Read the model definition and answer for the solid it produces. Units are mm, in the model's axes. A direction names the side the tool comes from. Give positions to 0.01 mm unless a question says otherwise; leave off trailing zeros. Write each loop counter-clockwise with the first axis right and the second up, starting at its lowest first coordinate (ties: lowest second). Pieces come first, ordered by that corner, then holes. Notation, with made-up numbers: (25.5, 14.5) -> (49.5, 14.5) arc R16 ccw to (49.5, 41.5) -> close; hole circle Ø10 at (31.25, -38). An arc over 180 degrees is marked (long way). Use a Markdown table: item, result.
from build123d import *

# Parameters (mm, degrees)
ESQUISSE14_W       = 64.629945491
ESQUISSE14_H       = 40
ESQUISSE14_R       = 1.719219897
ESQUISSE14_R_2     = 0.762879998
BOSS_EXTRU_1_DEPTH = 2
ESQUISSE15_W       = 64.629945491
ESQUISSE15_H       = 4
BOSS_EXTRU_2_DEPTH = 10


with BuildPart() as part:
    # Esquisse14 → Boss.-Extru.1 (new body)
    with BuildSketch(Plane.XY):
        with Locations((-35.198967366, -21.902230173)):
            Rectangle(ESQUISSE14_W, ESQUISSE14_H)
        with Locations((-10.253804476, -19.851102207)):
            Circle(ESQUISSE14_R, mode=Mode.SUBTRACT)
        with Locations((-9.464985935, -35.965799335)):
            Circle(ESQUISSE14_R, mode=Mode.SUBTRACT)
        with Locations((-58.998745092, -18.695161475)):
            Circle(ESQUISSE14_R, mode=Mode.SUBTRACT)
        with Locations((-60.03027703, -35.965799335)):
            Circle(ESQUISSE14_R, mode=Mode.SUBTRACT)
        with Locations((-11.973024373, -22.81882365)):
            Circle(ESQUISSE14_R_2, mode=Mode.SUBTRACT)
    extrude(amount=-BOSS_EXTRU_1_DEPTH)

    # Esquisse15 → Boss.-Extru.2 (add)
    with BuildSketch(Plane.XY):
        with Locations((-35.198967366, -10.343644154)):
            Rectangle(ESQUISSE15_W, ESQUISSE15_H)
    extrude(amount=BOSS_EXTRU_2_DEPTH)


solid = part.part
Item 1: A cutting plane is placed at C-C (y = -29). Give the vertices of the cut face in (x, z).
Return value:
| item | result |
|---|---|
| outline | (-67.51, -2) -> (-2.88, -2) -> (-2.88, 0) -> (-67.51, 0) -> close |
Item 2: A cutting plane is placed at B-B (x = -60). Give the vertices of the cut face in (y, z).
Return value:
| item | result |
|---|---|
| outline | (-41.9, -2) -> (-37.68, -2) -> (-37.68, 0) -> (-41.9, 0) -> close; (-34.25, -2) -> (-20.09, -2) -> (-20.09, 0) -> (-34.25, 0) -> close; (-17.3, -2) -> (-1.9, -2) -> (-1.9, 0) -> (-8.34, 0) -> (-8.34, 10) -> (-12.34, 10) -> (-12.34, 0) -> (-17.3, 0) -> close |
Item 3: A cutting plane is placed at A-A (x = -41.5). Give the vertices of the cut face in (y, z).
Return value:
| item | result |
|---|---|
| outline | (-41.9, -2) -> (-1.9, -2) -> (-1.9, 0) -> (-8.34, 0) -> (-8.34, 10) -> (-12.34, 10) -> (-12.34, 0) -> (-41.9, 0) -> close |
Item 4: Each of these flat-tipped pins is pushed along its axis until it touches: P1, Ø1.8, axis at x = -11.97, y = -22.82, coming from the +Z side; P2, Ø1, axis at x = -38, z = 1.5, coming from the +Y side. Where does it stop, or does it pass through?
Return value:
| item | result |
|---|---|
| P1 | z = 0 |
| P2 | y = -8.34 |
Item 5: A tool of negligible diameter and unlimited length cuts with its end or side. For faces 1 (the face through (-36, -8.344, 5)), 2 (the face through (-36, -27, 0)), 3 (the face through (-11.52, -18.69, -0.99)), from which of +Z, -Z, +X, -X, +Y, -Y can it reach the whole face along a straight path? Write none if from no direction.
Return value:
| item | result |
|---|---|
| face 1 | +Z, +X, -X, +Y |
| face 2 | +Z, +X, -X, -Y |
| face 3 | +Z, -Z |
Item 6: A cutting plane is placed at D-D (z = 8). Give the vertices of the cut face in (x, y), then the cut area to 3 significant figures.
Return value:
| item | result |
|---|---|
| outline | (-67.51, -12.34) -> (-2.88, -12.34) -> (-2.88, -8.34) -> (-67.51, -8.34) -> close |
| area | 259 mm^2 |
Item 7: Straight lines are drawn through the part: line 1 along Y through (x, z) = (-31, 2.25); line 2 along Z through (x, y) = (-46, -30). For each, find the intervals that lie inside material, in ascending order. Write a range as [from, to].
Return value:
| item | result |
|---|---|
| line 1 | [-12.34, -8.34] |
| line 2 | [-2, 0] |
Item 8: For a pull along Y with two mould halves and no side action, classify faces 4 (the face through (-36, -5, 0)), 5 (the face through (-36, -12.344, 5)), 6 (the face through (-7.877, -36.624, -0.986)) as +Y half, -Y half, draft (parallel to the pull), parting line (faces both ways), or undercut.
Return value:
| item | result |
|---|---|
| face 4 | draft |
| face 5 | -Y half |
| face 6 | undercut |
